Read the model definition and answer for the solid it produces. Units are mm, in the model's axes. Coordinates: 2 decimals unless noted, no trailing zeros. Order: outer loops, then holes, each group sorted by start corner. A loop starts at its lowest first (then second) coordinate and runs counter-clockwise, first axis right, second up.
```python
from build123d import *

# Parameters (mm, degrees)
SKETCH1_W           = 700
SKETCH1_H           = 350
BOSS_EXTRUDE2_DEPTH = 5
SKETCH2_R           = 15
SKETCH2_R_2         = 10
CUT_EXTRUDE1_DEPTH  = 10
FILLET1_R           = 35
SKETCH3_W           = 140
SKETCH3_H           = 140
CUT_EXTRUDE2_DEPTH  = 789.23060426
CHAMFER1_SIZE       = 50
CHAMFER1_SIZE2      = 36.602540378


with BuildPart() as part:
    # Sketch1 → Boss-Extrude2 (new, symmetric)
    with BuildSketch(Plane.XY):
        Polygon((350, -175), (-350, -175), (480.560796608, -397.548094716), (680.560796608, -397.548094716), (350, 175), align=None)
        Rectangle(SKETCH1_W, SKETCH1_H)
    extrude(amount=BOSS_EXTRUDE2_DEPTH, both=True)

    # Sketch2 → Cut-Extrude1 (cut)
    with BuildSketch(Plane.XY.offset(5)):
        with Locations((-320, 150)):
            Circle(SKETCH2_R)
        with Locations((180, 150)):
            Circle(SKETCH2_R_2)
    extrude(amount=-CUT_EXTRUDE1_DEPTH, mode=Mode.SUBTRACT)

    # Fillet1
    fillet1_edges = [part.edges().sort_by_distance(p)[0] for p in [
        (-350, 175, 0),
    ]]
    fillet(fillet1_edges, radius=FILLET1_R)

    # Sketch3 → Cut-Extrude2 (cut, through all)
    with BuildSketch(Plane.XY.offset(5)):
        with Locations((-280, -90)):
            Rectangle(SKETCH3_W, SKETCH3_H)
        Polygon((225.111069989, 157.48711306), (225.111069989, -128.301270189), (525.111069989, -128.301270189), (360.111069989, 157.48711306), align=None)
    extrude(amount=-CUT_EXTRUDE2_DEPTH, mode=Mode.SUBTRACT)

    # Chamfer1
    chamfer1_edges = [part.edges().sort_by_distance(p)[0] for p in [
        (680.560796608, -397.548094716, 0),
    ]]
    chamfer1_side = [part.faces().sort_by_distance(p)[0] for p in [
        (580.560796608, -397.548094716, 0),
    ]]
    chamfer(chamfer1_edges, length=CHAMFER1_SIZE, length2=CHAMFER1_SIZE2, reference=chamfer1_side[0])


solid = part.part
```
1) Straight lines are drawn through the part: line 1 (Y direction, x = -320, z = 0); line 2 (X direction, y = -63.5, z = 4); line 3 (Y direction, x = 298, z = -4.25). For each, find the intervals that lie inside material, in ascending order.
A:
line 1: y = -183.04 to -160, -20 to 135, 165 to 174.64
line 2: x = -210 to 225.11
line 3: y = -348.63 to -128.3, 157.49 to 175
2) Determine the mould class of faces 1 (the cylindrical face through (-306.144, 144.255, 0.07)), 2 (the cylindrical face through (189.237, 146.17, 0.07)), 3 (the flat face through (37, -107, -5)), 4 (the flat face through (646.63, -381.48, -0.07)) for opening direction X: pulls with the +X half, pulls with the -X half, needs draft (parallel to the pull), parting line crosses it, or undercut.
A:
face 1: undercut
face 2: undercut
face 3: needs draft
face 4: pulls with the +X half
3) A cutting plane is placed at A-A, the plane z = -0.25. Determine the outline of the cut face in (x, y).
A:
outline: (-350, -175) - (480.56, -397.55) - (630.56, -397.55) - (662.26, -365.85) - (525.11, -128.3) - (225.11, -128.3) - (225.11, 157.49) - (360.11, 157.49) - (350, 175) - (-315, 175) arc R35 ccw to (-350, 140) - (-350, -20) - (-210, -20) - (-210, -160) - (-350, -160) - close; hole circle Ø30 at (-320, 150); hole circle Ø20 at (180, 150)
4) Flat-ended cylindrical pins translate along their axes: pin 1 Ø24 at (x, y) = (-320, 150) entering from -Z; pin 2 Ø5 at (x, z) = (-162, -2.5) entering from -Y; pin 3 Ø3 at (x, z) = (-266, 2.5) entering from -Y; pin 4 Ø4 at (x, z) = (267.5, 3) entering from -Y. Find the tip coordinate at first contact, or state that the pin passes through.
A:
pin 1: passes through
pin 2: stops at y = -226.04
pin 3: stops at y = -197.91
pin 4: stops at y = -340.99
5) A cutting plane is placed at B-B, the plane x = 180. Determine the outline of the cut face in (y, z).
A:
outline: (-317.01, -5) - (140, -5) - (140, 5) - (-317.01, 5) - close; (160, -5) - (175, -5) - (175, 5) - (160, 5) - close
6) A cutting plane is placed at D-D, the plane x = 285. Determine the outline of the cut face in (y, z).
A:
outline: (-345.15, -5) - (-128.3, -5) - (-128.3, 5) - (-345.15, 5) - close; (157.49, -5) - (175, -5) - (175, 5) - (157.49, 5) - close
7) A cutting plane is placed at C-C, the plane y = -57.5. Determine the outline of the cut face in (x, z), and give its area (3 significant figures).
A:
outline: (-210, -5) - (225.11, -5) - (225.11, 5) - (-210, 5) - close
area: 4,350 mm2
